```python
from build123d import *

# Parameters (mm, degrees)
SKETCH_1_W               = 300
SKETCH_1_H               = 300
EXTRUDE_1_DEPTH          = 3
FILLET_1_R               = 10
SKETCH_2_R               = 5
CUT_EXTRUDE_1_DEPTH      = 213.153246499
MIRROR_2_COPY_1_SKETCH_R = 5
MIRROR_2_COPY_1_DEPTH    = 213.153246499
SKETCH_3_R               = 5
CUT_EXTRUDE_2_DEPTH      = 213.153246499
SKETCH_4_R               = 5
CUT_EXTRUDE_3_DEPTH      = 213.153246499


with BuildPart() as part:
    # 草图1 → 凸台-拉伸1 (new body)
    with BuildSketch(Plane(origin=(0, 0, 0), x_dir=(1, 0, 0), z_dir=(0, 1, 0))):
        Rectangle(SKETCH_1_W, SKETCH_1_H)
    extrude(amount=EXTRUDE_1_DEPTH)

    # 圆角1
    fillet_1_edges = [part.edges().sort_by_distance(p)[0] for p in [
        (-150, 1.5, -150),
        (150, 1.5, -150),
        (150, 1.5, 150),
        (-150, 1.5, 150),
    ]]
    fillet(fillet_1_edges, radius=FILLET_1_R)

    # 草图2 → 切除-拉伸1 (cut, through all)
    with BuildSketch(Plane(origin=(0, 3, 0), x_dir=(1, 0, 0), z_dir=(0, 1, 0))):
        with Locations(Location((-130, 130, 0), (0, 0, 270))):
            Circle(SKETCH_2_R)
    cut_extrude_1 = extrude(amount=-CUT_EXTRUDE_1_DEPTH, mode=Mode.SUBTRACT)

    # 镜向1: 切除-拉伸1 across plane
    add(cut_extrude_1.mirror(Plane.XY), mode=Mode.SUBTRACT)

    # 镜向2: 切除-拉伸1 across plane
    add(cut_extrude_1.mirror(Plane(origin=(0, 0, 0), x_dir=(0, 0, 1), z_dir=(1, 0, 0))), mode=Mode.SUBTRACT)

    # 镜向2 copy 1 sketch → 镜向2 copy 1 (cut, through all)
    with BuildSketch(Plane(origin=(0, 3, 0), x_dir=(-1, 0, 0), z_dir=(0, 1, 0))):
        with Locations(Location((-130, 130, 0), (0, 0, 270))):
            Circle(MIRROR_2_COPY_1_SKETCH_R)
    extrude(amount=-MIRROR_2_COPY_1_DEPTH, mode=Mode.SUBTRACT)

    # 草图3 → 切除-拉伸2 (cut, through all)
    with BuildSketch(Plane(origin=(0, 3, 0), x_dir=(1, 0, 0), z_dir=(0, 1, 0))):
        with Locations(Location((-130, 0, 0), (0, 0, 270))):
            Circle(SKETCH_3_R)
    cut_extrude_2 = extrude(amount=-CUT_EXTRUDE_2_DEPTH, mode=Mode.SUBTRACT)

    # 镜向3: 切除-拉伸2 across plane
    add(cut_extrude_2.mirror(Plane(origin=(0, 0, 0), x_dir=(0, 0, 1), z_dir=(1, 0, 0))), mode=Mode.SUBTRACT)

    # 草图4 → 切除-拉伸3 (cut, through all)
    with BuildSketch(Plane(origin=(0, 3, 0), x_dir=(1, 0, 0), z_dir=(0, 1, 0))):
        with Locations(Location((0, 130, 0), (0, 0, 270))):
            Circle(SKETCH_4_R)
        with Locations(Location((0, -130, 0), (0, 0, 270))):
            Circle(SKETCH_4_R)
    extrude(amount=-CUT_EXTRUDE_3_DEPTH, mode=Mode.SUBTRACT)


solid = part.part
```
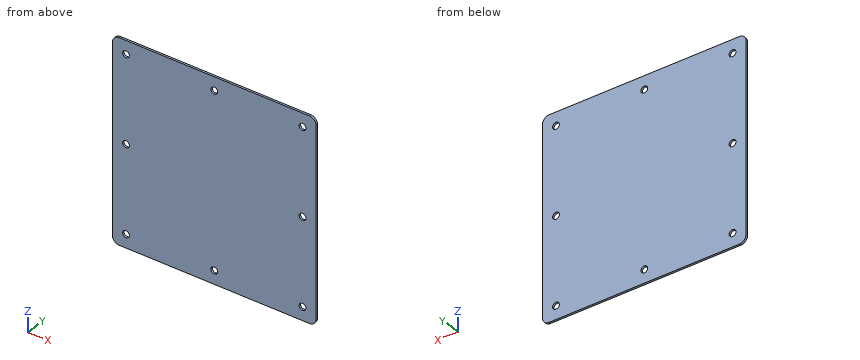
The model under review builds one solid part; all positions refer to its coordinate system, in mm. Coordinates: 2 decimals unless noted, no trailing zeros. Write each loop counter-clockwise with the first axis right and the second up, starting at its lowest first coordinate (ties: lowest second). Pieces come first, ordered by that corner, then holes.
1) We need section C-C on x = 130. State the section outline as (y, z) points, then the cut area to 3 significant figures.
2) We need section A-A on z = 0. State the section outline as (x, y) points, then the cut area to 3 significant figures.
3) We need section D-D on z = -130. State the section outline as (x, y) points, then the cut area to 3 significant figures.
4) We need section B-B on x = 0. State the section outline as (y, z) points, then the cut area to 3 significant figures.
5) To check wall thickness, follow probe 1 along X at (y, z) = (0.7, -130). State the ranges of the line that lie inside material, in increasing order.
Answer list:
1. outline: (0, -150) - (3, -150) - (3, -135) - (0, -135) - close; (0, -125) - (3, -125) - (3, -5) - (0, -5) - close; (0, 5) - (3, 5) - (3, 125) - (0, 125) - close; (0, 135) - (3, 135) - (3, 150) - (0, 150) - close
1. area: 810 mm2
2. outline: (-150, 0) - (-135, 0) - (-135, 3) - (-150, 3) - close; (-125, 0) - (125, 0) - (125, 3) - (-125, 3) - close; (135, 0) - (150, 0) - (150, 3) - (135, 3) - close
2. area: 840 mm2
3. outline: (-150, 0) - (-135, 0) - (-135, 3) - (-150, 3) - close; (-125, 0) - (-5, 0) - (-5, 3) - (-125, 3) - close; (5, 0) - (125, 0) - (125, 3) - (5, 3) - close; (135, 0) - (150, 0) - (150, 3) - (135, 3) - close
3. area: 810 mm2
4. outline: (0, -150) - (3, -150) - (3, -135) - (0, -135) - close; (0, -125) - (3, -125) - (3, 125) - (0, 125) - close; (0, 135) - (3, 135) - (3, 150) - (0, 150) - close
4. area: 840 mm2
5. probe 1: x = -150 to -135, -125 to -5, 5 to 125, 135 to 150
